Read the model definition and answer for the solid it produces. Units are mm, in the model's axes. A direction names the side the tool comes from. Give positions to 0.01 mm unless a question says otherwise; leave off trailing zeros. Write each loop counter-clockwise with the first axis right and the second up, starting at its lowest first coordinate (ties: lowest second). Pieces come first, ordered by that corner, then holes. Notation, with made-up numbers: M -38.75,78 L -3.75,78 A16 ccw -3.75,92 Z; hole C 50,13 d8. An arc over 180 degrees is marked long. Put each result on its own line as item: value.
from build123d import *

# Parameters (mm, degrees)
SKETCH_1_W          = 250
SKETCH_1_H          = 250
EXTRUDE_1_DEPTH     = 2
SKETCH_2_W          = 250
SKETCH_2_H          = 125
CUT_EXTRUDE_1_DEPTH = 2
SKETCH_6_W          = 10
SKETCH_6_H          = 10
EXTRUDE_3_DEPTH     = 10
CUT_EXTRUDE_2_DEPTH = 178.059312096


with BuildPart() as part:
    # 草图1 → 凸台-拉伸1 (new body)
    with BuildSketch(Plane(origin=(0, 0, 0), x_dir=(1, 0, 0), z_dir=(0, 1, 0))):
        Rectangle(SKETCH_1_W, SKETCH_1_H)
    extrude(amount=EXTRUDE_1_DEPTH)

    # 草图2 → 切除-拉伸1 (cut)
    with BuildSketch(Plane(origin=(0, 2, 0), x_dir=(1, 0, 0), z_dir=(0, 1, 0))):
        with Locations((0, -62.5)):
            Rectangle(SKETCH_2_W, SKETCH_2_H)
    extrude(amount=-CUT_EXTRUDE_1_DEPTH, mode=Mode.SUBTRACT)

    # 草图6 → 凸台-拉伸3 (add)
    with BuildSketch(Plane.XZ):
        with Locations((-105.253353702, -19.703268914)):
            Rectangle(SKETCH_6_W, SKETCH_6_H)
        with Locations((-105.253353702, -104.703268914)):
            Rectangle(SKETCH_6_W, SKETCH_6_H)
        with Locations((104.746646298, -19.703268914)):
            Rectangle(SKETCH_6_W, SKETCH_6_H)
        with Locations((104.746646298, -104.703268914)):
            Rectangle(SKETCH_6_W, SKETCH_6_H)
    extrude(amount=EXTRUDE_3_DEPTH)

    # 草图7 → 切除-拉伸2 (cut, through all)
    with BuildSketch(Plane(origin=(0, 0, -125), x_dir=(-1, 0, 0), z_dir=(0, 0, -1))):
        Polygon((-125, 2), (-125, 0), (-121.535898385, 2), align=None)
        Polygon((121.535898385, 2), (125, 2), (125, 0), align=None)
    extrude(amount=-CUT_EXTRUDE_2_DEPTH, mode=Mode.SUBTRACT)


solid = part.part
(1) Given pin 1 Ø3 at (x, y) = (-104.5, -4) entering from +Z; pin 2 Ø5 at (y, z) = (-4, -104.5) entering from +X; pin 3 Ø3 at (x, y) = (107, -3) entering from -Z; pin 4 Ø6 at (y, z) = (-4, -95.5) entering from -X, each flat-ended and moving along its own axis, determine where each tip first touches the part or whether it passes through.
Result:
pin 1: stops at z = -14.7
pin 2: stops at x = 109.75
pin 3: stops at z = -109.7
pin 4: passes through
(2) Section A-A on y = -3.25 is taken. Determine the outline of the cut face in (x, z).
Result:
outline: M -110.25,-109.7 L -100.25,-109.7 L -100.25,-99.7 L -110.25,-99.7 Z; M -110.25,-24.7 L -100.25,-24.7 L -100.25,-14.7 L -110.25,-14.7 Z; M 99.75,-109.7 L 109.75,-109.7 L 109.75,-99.7 L 99.75,-99.7 Z; M 99.75,-24.7 L 109.75,-24.7 L 109.75,-14.7 L 99.75,-14.7 Z
(3) For a pull along Z with two mould halves and no side action, classify faces 5 (the face through (105, -5, -24.703)), 6 (the face through (-105, -5, -109.703)), 7 (the face through (-100.253, -5, -20)) as +Z half, -Z half, draft (parallel to the pull), parting line (faces both ways), or undercut.
Result:
face 5: undercut
face 6: -Z half
face 7: draft
(4) Which of the six approach directions +Z, -Z, +X, -X, +Y, -Y give full straight-line access (tool end or side, diameter ignored) to faces 1 (the face through (-110.253, -5, -105)), 2 (the face through (-105, -5, -24.703)), 3 (the face through (99.747, -5, -20)), 4 (the face through (105, -5, -109.703))?
Result:
face 1: +Z, -Z, -X, -Y
face 2: +X, -X, -Y
face 3: +Z, -Z, -Y
face 4: -Z, +X, -X, -Y
(5) Section D-D on z = -74.5 is taken. Determine the outline of the cut face in (x, y).
Result:
outline: M -125,0 L 125,0 L 121.54,2 L -121.54,2 Z
(6) Section C-C on x = 1 is taken. Determine the outline of the cut face in (y, z), and give its area (3 significant figures).
Result:
outline: M 0,-125 L 2,-125 L 2,0 L 0,0 Z
area: 250 mm²
(7) Straight lines are drawn through the part: line 1 along Z through (x, y) = (-108.5, -1); line 2 along X through (y, z) = (-2.75, -24.5); line 3 along Y through (x, z) = (61.5, -27). For each, find the intervals that lie inside material, in ascending order. Write a range as from..to.
Result:
line 1: z = -109.7..-99.7, -24.7..-14.7
line 2: x = -110.25..-100.25, 99.75..109.75
line 3: y = 0..2
(8) Section B-B on z = -22 is taken. Determine the outline of the cut face in (x, y).
Result:
outline: M -125,0 L -110.25,0 L -110.25,-10 L -100.25,-10 L -100.25,0 L 99.75,0 L 99.75,-10 L 109.75,-10 L 109.75,0 L 125,0 L 121.54,2 L -121.54,2 Z
